Work out the finished part from the listing and answer in its coordinate system (mm). Coordinates: 2 decimals unless noted, no trailing zeros. Order: outer loops, then holes, each group sorted by start corner. A loop starts at its lowest first (then second) coordinate and runs counter-clockwise, first axis right, second up.
1. The part is cut by section A-A, the plane x = 0. Give the vertices of the cut face in (y, z), then the cut area to 3 significant figures.
2. The part is cut by section C-C, the plane z = 18. Give the vertices of the cut face in (x, y).
3. Find the intervals of material crossed by probe 1 along X at (y, z) = (0, 39); probe 2 along X at (y, z) = (-0.5, 7.5), in increasing order.
4. The part is cut by section B-B, the plane y = 0. Give the vertices of the cut face in (x, z), then the cut area to 3 significant figures.
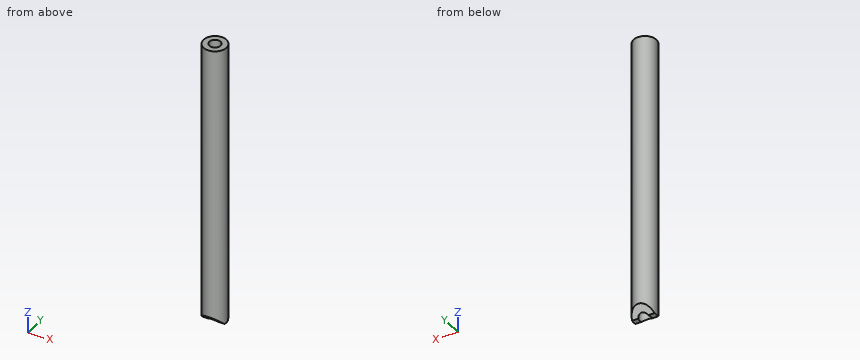
```python
from build123d import *

# Parameters (mm, degrees)
SKETCH089_R          = 2
SKETCH089_R_2        = 1
PAD030_DEPTH         = 50
POCKET025_DEPTH      = 2.001
POCKET025_DEPTH_BACK = -2.001


with BuildPart() as part:
    # Sketch089 → Pad030 (new body)
    with BuildSketch(Plane.XY):
        Circle(SKETCH089_R)
        Circle(SKETCH089_R_2, mode=Mode.SUBTRACT)
    extrude(amount=PAD030_DEPTH)

    # Sketch090 → Pocket025 (cut, two sides)
    with BuildSketch(Plane.YZ) as pocket025_sk:
        Polygon((0, -0.5), (4, 3.5), (4, -3.5), (-4, -3.5), (-4, 3.5), align=None)
    extrude(amount=-POCKET025_DEPTH, mode=Mode.SUBTRACT)
    extrude(pocket025_sk.sketch, amount=-POCKET025_DEPTH_BACK, mode=Mode.SUBTRACT)


solid = part.part
```
Geometry says:
1. outline: (-2, 1.5) - (-1, 0.5) - (-1, 50) - (-2, 50) - close; (1, 0.5) - (2, 1.5) - (2, 50) - (1, 50) - close
1. area: 98.0 mm2
2. outline: circle Ø4 at (0, 0); hole circle Ø2 at (0, 0)
3. probe 1: x = -2 to -1, 1 to 2
3. probe 2: x = -1.94 to -0.87, 0.87 to 1.94
4. outline: (-2, 0) - (-1, 0) - (-1, 50) - (-2, 50) - close; (1, 0) - (2, 0) - (2, 50) - (1, 50) - close
4. area: 100 mm2
